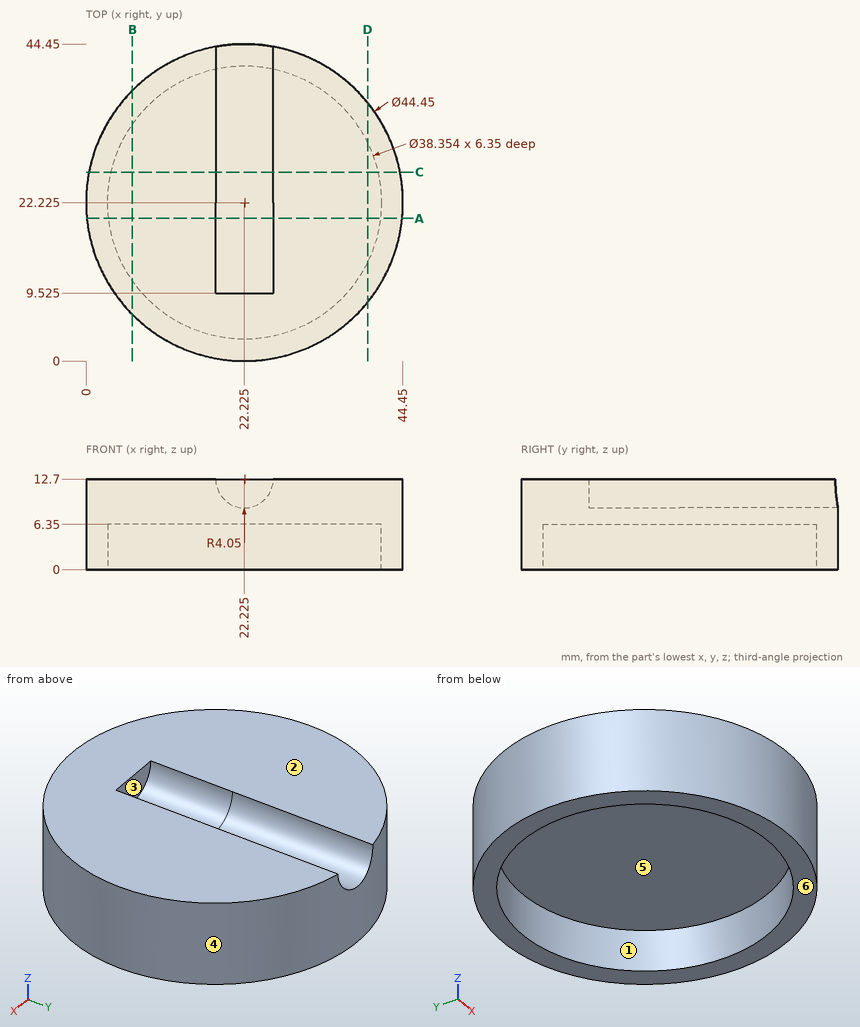
Here's the drawing with two shaded views (mm, measured from the low corner). I have some questions. A direction names the side the tool comes from. Give positions to 0.01 mm unless a question says otherwise; leave off trailing zeros. Loops run counter-clockwise (first coordinate to the right, second up) from the corner with the lowest first, then second, coordinate; pieces in that order, holes last. Notation, with made-up numbers: (-10, -3.5) - (2, -3.5) arc R10 ccw to (2, 1.5) - close; hole circle Ø11 at (86, 69.5). An arc over 180 degrees is marked (long way). One line per item, written item: value.
(1) If we section it at A-A, the plane y = 20: List the corners of the cut face in (x, z) for me (3 decimals).
Verdict:
outline: (0.112, 0) - (3.178, 0) - (3.178, 6.35) - (41.272, 6.35) - (41.272, 0) - (44.338, 0) - (44.338, 12.7) - (26.275, 12.7) arc R4.05 cw to (18.175, 12.7) - (0.112, 12.7) - close
(2) If we section it at B-B, the plane x = 6.5: List the corners of the cut face in (y, z) for me, plus the area to 3 significant figures.
Verdict:
outline: (6.52, 0) - (11.25, 0) - (11.25, 6.35) - (33.2, 6.35) - (33.2, 0) - (37.93, 0) - (37.93, 12.7) - (6.52, 12.7) - close
area: 260 mm^2
(3) On a 3-axis mill with a long thin cutter (end or side, diameter ignored), from which of +Z, -Z, +X, -X, +Y, -Y can I reach the whole of each face in a straight line? I mean the marked faces 5 and 6. Say none if no direction works.
Verdict:
face 5: -Z
face 6: -Z, +X, -X, +Y, -Y
(4) If we section it at C-C, the plane y = 26.5: List the corners of the cut face in (x, z) for me (3 decimals), plus the area to 3 significant figures.
Verdict:
outline: (0.415, 0) - (3.531, 0) - (3.531, 6.35) - (40.919, 6.35) - (40.919, 0) - (44.035, 0) - (44.035, 12.7) - (26.275, 12.7) arc R4.05 cw to (18.175, 12.7) - (0.415, 12.7) - close
area: 291 mm^2
(5) If we section it at D-D, the plane x = 39.5: List the corners of the cut face in (y, z) for me.
Verdict:
outline: (8.24, 0) - (13.9, 0) - (13.9, 6.35) - (30.55, 6.35) - (30.55, 0) - (36.21, 0) - (36.21, 12.7) - (8.24, 12.7) - close
(6) I need wall thicknesses on line 1 along Y through (x, z) = (22, 1.25); line 2 along Y through (x, z) = (10.5, 3.25); line 3 along Z through (x, y) = (17.5, 16.5). Which ranges of each line are inside material? Lowest first, please.
Verdict:
line 1: 0 to 3.05, 41.4 to 44.45
line 2: 3.34 to 7.05, 37.4 to 41.11
line 3: 6.35 to 12.7
(7) If we mould it in two halves opening along X, with no side actions, what happens to the marked faces 1, 2, 3 and 4? For each: released by +X, released by -X, zero draft, split by the parting line, or undercut.
Verdict:
face 1: undercut
face 2: zero draft
face 3: undercut
face 4: split by the parting line
(8) I'm going to push flat-ended pins straight in: pin 1 (5 mm diameter, centred on x = 39.5, z = 8.5, fed in from -Y); pin 2 (1.5 mm diameter, centred on x = 24.5, y = 16, fed in from +Z); pin 3 (5 mm diameter, centred on x = 30, y = 35.5, fed in from -Z); pin 4 (4.5 mm diameter, centred on x = 21.5, z = 10, fed in from +Y). Where does each tip first touch, or does it pass through?
Verdict:
pin 1: y = 5.62
pin 2: z = 10.01
pin 3: z = 6.35
pin 4: y = 44.45
